Job drawing, mm, ordinate dimensions from the low corner. One solid piece. A direction names the side the tool comes from. Give positions to 0.01 mm unless a question says otherwise; leave off trailing zeros. Loops run counter-clockwise (first coordinate to the right, second up) from the corner with the lowest first, then second, coordinate; pieces in that order, holes last. Notation, with made-up numbers: M 17,57.5 L 72,57.5 A38 ccw 72,96.5 Z; hole C 28.5,-3 d6. An arc over 180 degrees is marked long. Answer in a Markdown table with one row per item.
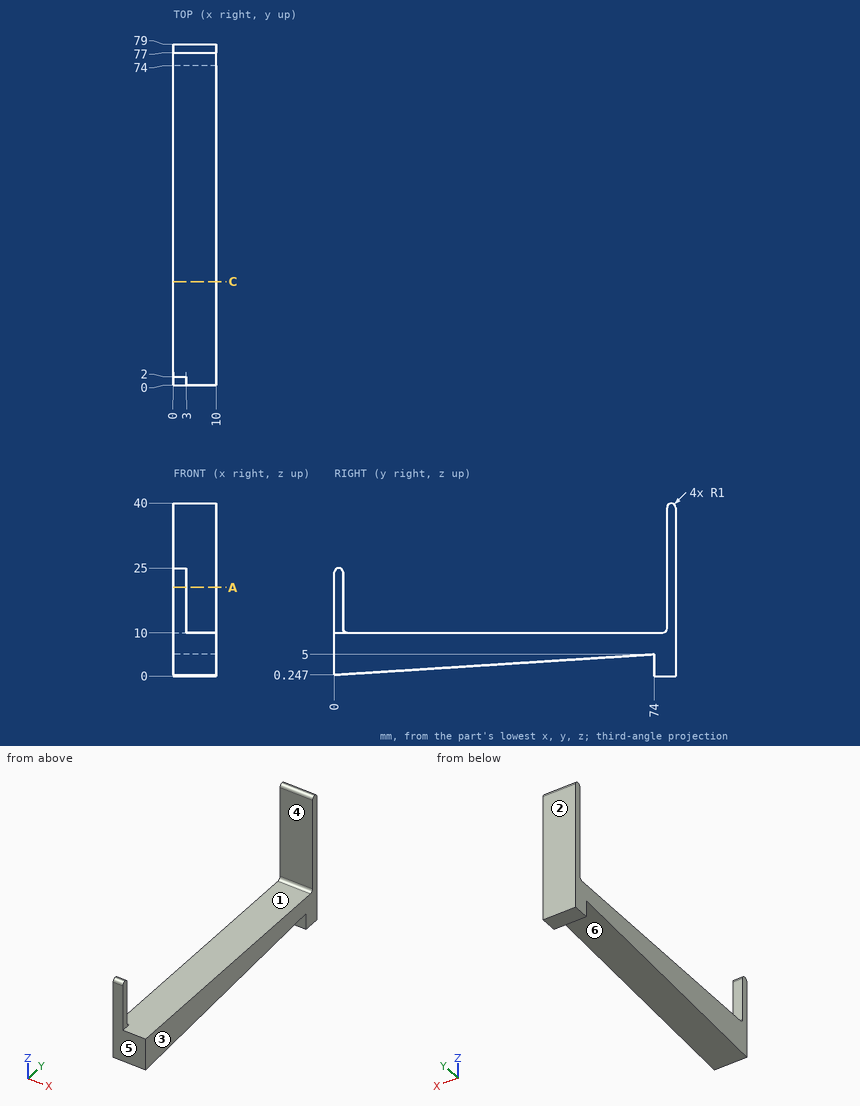
(1) Saw through at A-A (z = 20.5). Write the cut outline in (x, y), plus the area to 3 significant figures.
Recorded:
| item | result |
|---|---|
| outline | M 0,0 L 3,0 L 3,2 L 0,2 Z; M 0,77 L 10,77 L 10,79 L 0,79 Z |
| area | 26.0 mm^2 |
(2) Which spindle directions (+Z, -Z, +X, -X, +Y, -Y) get a long thin tool onto all of the face, cutting with end or side? Do the marked faces 5 and 6. Say none if no direction does.
Recorded:
| item | result |
|---|---|
| face 5 | +Z, -Z, +X, -X, -Y |
| face 6 | -Z, +X, -X |
(3) Drill centre lines: line 1 along Y through (x, z) = (2.75, 23.5); line 2 along Y through (x, z) = (2, 35); line 3 along Z through (x, y) = (4.25, 32). Where is each one in solid material? Low to high.
Recorded:
| item | result |
|---|---|
| line 1 | y = 0 to 2, 77 to 79 |
| line 2 | y = 77 to 79 |
| line 3 | z = 2.3 to 10 |
(4) Saw through at C-C (y = 24). Write the cut outline in (x, z).
Recorded:
| item | result |
|---|---|
| outline | M 0,1.79 L 10,1.79 L 10,10 L 0,10 Z |
(5) Pull direction Y, two halves, no side cores. Call the marked faces 1, 2, 3 and 4: +Y half, -Y half, draft (parallel to the pull), parting line (faces both ways), or undercut.
Recorded:
| item | result |
|---|---|
| face 1 | undercut |
| face 2 | +Y half |
| face 3 | draft |
| face 4 | undercut |
(6) Pin check, flat tips, straight feed: pin 1 Ø5 at (x, y) = (5, 51) entering from +Z; pin 2 Ø5 at (x, y) = (2, 27.5) entering from -Z; pin 3 Ø5 at (x, y) = (1, 18) entering from -Z. Stop position of each tip, or through.
Recorded:
| item | result |
|---|---|
| pin 1 | stops at z = 10 |
| pin 2 | stops at z = 1.85 |
| pin 3 | stops at z = 1.24 |
